Source: CAD feature listing. Evaluate the final solid. Frame: model axes, mm. Face numbers are marked on the shaded views. A direction names the side the tool comes from. Round coordinates to 2 decimals unless told otherwise and drop trailing zeros. Loops run counter-clockwise (first coordinate to the right, second up) from the corner with the lowest first, then second, coordinate; pieces in that order, holes last. Notation, with made-up numbers: (14.25, -9.5) -> (56.25, -9.5) arc R26 ccw to (56.25, 8.5) -> close; hole circle Ø9 at (26, 19). An arc over 180 degrees is marked (long way). Return JSON: item names as keys, results as strings. Group by question number.
```python
from build123d import *

# Parameters (mm, degrees)
SKETCH_1_R          = 4
EXTRUDE_1_DEPTH     = 8
SKETCH_3_R          = 6
EXTRUDE_2_DEPTH     = 2
SKETCH_2_R          = 1.35
CUT_EXTRUDE_1_DEPTH = 12


with BuildPart() as part:
    # 스케치1 → 보스-돌출1 (new body)
    with BuildSketch(Plane(origin=(0, 0, 0), x_dir=(1, 0, 0), z_dir=(0, 1, 0))):
        Circle(SKETCH_1_R)
    extrude(amount=EXTRUDE_1_DEPTH)

    # 스케치3 → 보스-돌출2 (add)
    with BuildSketch(Plane.XZ):
        Circle(SKETCH_3_R)
    extrude(amount=EXTRUDE_2_DEPTH)

    # 스케치2 → 컷-돌출1 (cut)
    with BuildSketch(Plane(origin=(0, 8, 0), x_dir=(1, 0, 0), z_dir=(0, 1, 0))):
        Circle(SKETCH_2_R)
    extrude(amount=-CUT_EXTRUDE_1_DEPTH, mode=Mode.SUBTRACT)


solid = part.part
```
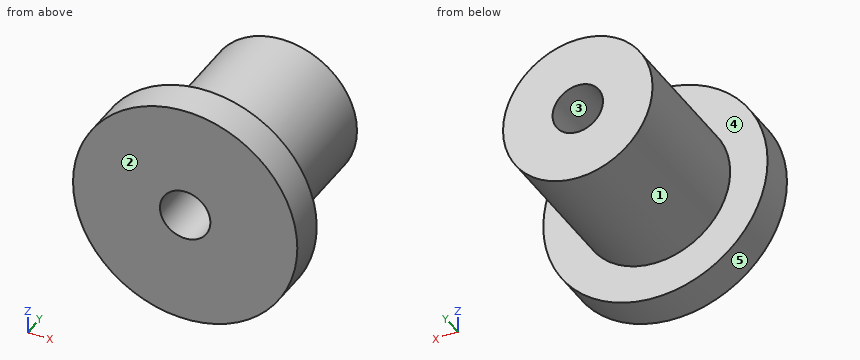
(1) Ray query, line 1 (Z direction, x = 0, y = 4); line 2 (Y direction, x = 4, z = -3.75). Return the intervals inside material, ascending.
(2) Cut plane B-B (y = 3). Return loops of the section in (x, z).
(3) Pin query (flat end, axial travel): pin 1 (5 mm diameter, centred on x = -2.5, y = 1, fed in from -Z); pin 2 (5 mm diameter, centred on x = -2.5, y = 3.5, fed in from -Z); pin 3 (1.5 mm diameter, centred on y = 0.5, z = -4.5, fed in from -X). Return the tip coordinate at first contact, or that it passes through.
(4) Cut plane A-A (x = 0). Return loops of the section in (y, z).
(5) Mould query, pull axis Z, two halves, no side actions, for the marked faces 1, 2 and 3. Classes: released by +Z, released by -Z, zero draft, split by the parting line, or undercut.
(6) Cut plane C-C (z = 1.75). Return loops of the section in (x, y), and give its area (3 significant figures).
(7) Set-up query: the marked faces 4 and 5. Return all of +Z, -Z, +X, -X, +Y, -Y with unobstructed straight access to the full face (end or side cutting, diameter ignored); none if empty.
(8) Cut plane D-D (x = -2.25). Return loops of the section in (y, z).
Answers follow:
{
 "1": {"line 1": "-4 to -1.35, 1.35 to 4", "line 2": "-2 to 0"},
 "2": {"outline": "circle Ø8 at (0, 0); hole circle Ø2.7 at (0, 0)"},
 "3": {"pin 1": "z = -6", "pin 2": "z = -4", "pin 3": "x = -4.52"},
 "4": {"outline": "(-2, -6) -> (0, -6) -> (0, -4) -> (8, -4) -> (8, -1.35) -> (-2, -1.35) -> close; (-2, 1.35) -> (8, 1.35) -> (8, 4) -> (0, 4) -> (0, 6) -> (-2, 6) -> close"},
 "5": {"face 1": "split by the parting line", "face 2": "zero draft", "face 3": "undercut"},
 "6": {"outline": "(-5.74, -2) -> (5.74, -2) -> (5.74, 0) -> (3.6, 0) -> (3.6, 8) -> (-3.6, 8) -> (-3.6, 0) -> (-5.74, 0) -> close", "area": "80.5 mm^2"},
 "7": {"face 4": "+Y", "face 5": "+Y, -Y"},
 "8": {"outline": "(-2, -5.56) -> (0, -5.56) -> (0, -3.31) -> (8, -3.31) -> (8, 3.31) -> (0, 3.31) -> (0, 5.56) -> (-2, 5.56) -> close"}
}
